from build123d import *

# Parameters (mm, degrees)
SKETCH1_R           = 37
BOSS_EXTRUDE1_DEPTH = 3
SKETCH1_3_R         = 30
SKETCH1_3_R_2       = 28
BOSS_EXTRUDE2_DEPTH = 29
SKETCH2_R           = 4
SKETCH2_R_2         = 2
CUT_EXTRUDE1_DEPTH  = 59.429444632


with BuildPart() as part:
    # Sketch1 → Boss-Extrude1 (new body)
    with BuildSketch(Plane(origin=(0, 0, 0), x_dir=(1, 0, 0), z_dir=(0, 1, 0))):
        with Locations(Location((0, 0, 0), (0, 0, 270))):
            Circle(SKETCH1_R)
    extrude(amount=BOSS_EXTRUDE1_DEPTH)

    # Sketch1_3 → Boss-Extrude2 (add)
    with BuildSketch(Plane(origin=(0, 0, 0), x_dir=(1, 0, 0), z_dir=(0, 1, 0))):
        with Locations(Location((0, 0, 0), (0, 0, 90))):
            Circle(SKETCH1_3_R)
        with Locations(Location((0, 0, 0), (0, 0, 90))):
            Circle(SKETCH1_3_R_2, mode=Mode.SUBTRACT)
    extrude(amount=BOSS_EXTRUDE2_DEPTH)

    # Sketch2 → Cut-Extrude1 (cut, through all)
    with BuildSketch(Plane(origin=(0, 3, 0), x_dir=(1, 0, 0), z_dir=(0, 1, 0))):
        with Locations(Location((0, 0, 0), (0, 0, 270))):
            Circle(SKETCH2_R)
        with Locations(Location((8, 0, 0), (0, 0, 270))):
            Circle(SKETCH2_R_2)
        with Locations(Location((0, -8, 0), (0, 0, 270))):
            Circle(SKETCH2_R_2)
        with Locations(Location((-8, 0, 0), (0, 0, 270))):
            Circle(SKETCH2_R_2)
        with Locations(Location((0, 8, 0), (0, 0, 270))):
            Circle(SKETCH2_R_2)
    extrude(amount=-CUT_EXTRUDE1_DEPTH, mode=Mode.SUBTRACT)


solid = part.part
Can you work these out from the model? Positions are in its coordinate system, mm. A direction names the side the tool comes from. Give positions to 0.01 mm unless a question says otherwise; leave off trailing zeros. Order: outer loops, then holes, each group sorted by start corner. A loop starts at its lowest first (then second) coordinate and runs counter-clockwise, first axis right, second up. Notation, with made-up numbers: M 83,31.25 L 101,31.25 A13 ccw 101,49.25 Z; hole C 9.25,54 d7. An arc over 180 degrees is marked long. Use a Markdown table: item, result. Add a question column.
Item 1: For faces 5 (the flat face through (0.4, 3, 5.8)), 6 (the flat face through (8, 0, -8)), which set-ups out of +Z, -Z, +X, -X, +Y, -Y let a thin tool reach every point of the face, with its end or its side?
Item 2: We'd pull the mould along Z, two halves only. Please class faces 1 (the cylindrical face through (-1.2, 1.5, -9.6)), 2 (the cylindrical face through (-6, 2, 0)), 3 (the flat face through (30.3, 3, -0.2)), 4 (the cylindrical face through (-14.17, 1.48, 34.18)): +Z half, -Z half, draft (parallel to the pull), parting line (faces both ways), or undercut.
Item 3: If I drill on L1, parallel to X at y = 2.1, z = 0; L2, parallel to X at y = 9, z = 0; L3, parallel to Y at x = -5, z = -8, over which ranges is the centre line in solid material (lowest first)? Write a range as [from, to].
Item 4: Suppose I cut it at D-D (z = -8). List the corners of the cut face in (x, y) for me.
Item 5: Will these pins go through, and if not, where does the flat tip stop? pin 1 (3 mm diameter, centred on x = 8, z = 0, fed in from -Y) (3 decimals); pin 2 (5 mm diameter, centred on y = 10.5, z = -9.5, fed in from -X); pin 3 (1.5 mm diameter, centred on y = 23.5, z = -10, fed in from -X); pin 4 (17 mm diameter, centred on x = 0.5, z = 2, fed in from +Y).
Item 6: Suppose I cut it at A-A (z = 0). List the corners of the cut face in (x, y) for me, then the cut area to 3 significant figures.
Item 7: Suppose I cut it at B-B (x = -8). List the corners of the cut face in (y, z) for me.
Item 8: Suppose I cut it at C-C (y = 26). List the corners of the cut face in (x, z) for me, then the cut area to 3 significant figures.
Answer sheet:
| question | item | result |
|---|---|---|
| 1 | face 5 | +Y |
| 1 | face 6 | +Z, -Z, +X, -X, -Y |
| 2 | face 1 | undercut |
| 2 | face 2 | undercut |
| 2 | face 3 | draft |
| 2 | face 4 | parting line |
| 3 | L1 | x = [-37, -10], [-6, -4], [4, 6], [10, 37] |
| 3 | L2 | x = [-30, -28], [28, 30] |
| 3 | L3 | y = [0, 3] |
| 4 | outline | M -36.12,0 L -2,0 L -2,3 L -26.83,3 L -26.83,29 L -28.91,29 L -28.91,3 L -36.12,3 Z; M 2,0 L 36.12,0 L 36.12,3 L 28.91,3 L 28.91,29 L 26.83,29 L 26.83,3 L 2,3 Z |
| 5 | pin 1 | passes through |
| 5 | pin 2 | stops at x = -29.17 |
| 5 | pin 3 | stops at x = -28.54 |
| 5 | pin 4 | stops at y = 3 |
| 6 | outline | M -37,0 L -10,0 L -10,3 L -28,3 L -28,29 L -30,29 L -30,3 L -37,3 Z; M -6,0 L -4,0 L -4,3 L -6,3 Z; M 4,0 L 6,0 L 6,3 L 4,3 Z; M 10,0 L 37,0 L 37,3 L 30,3 L 30,29 L 28,29 L 28,3 L 10,3 Z |
| 6 | area | 278 mm² |
| 7 | outline | M 0,-36.12 L 3,-36.12 L 3,-28.91 L 29,-28.91 L 29,-26.83 L 3,-26.83 L 3,-2 L 0,-2 Z; M 0,2 L 3,2 L 3,26.83 L 29,26.83 L 29,28.91 L 3,28.91 L 3,36.12 L 0,36.12 Z |
| 8 | outline | C 0,0 d60; hole C 0,0 d56 |
| 8 | area | 364 mm² |
